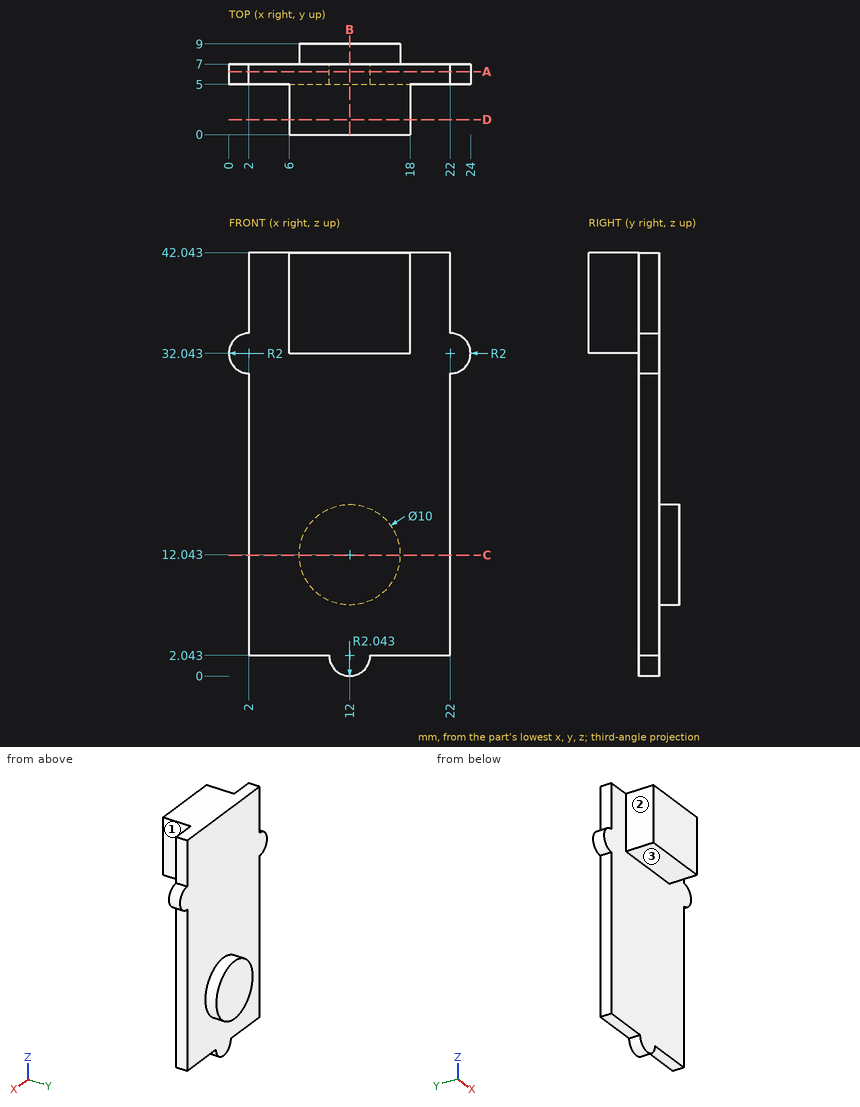
Input: dimensioned drawing with shaded views. Units: mm. Origin: part minimum x, y, z. A direction names the side the tool comes from. Give positions to 0.01 mm unless a question says otherwise; leave off trailing zeros. Loops run counter-clockwise (first coordinate to the right, second up) from the corner with the lowest first, then second, coordinate; pieces in that order, holes last. Notation, with made-up numbers: M -34.5,0.5 L -5.5,0.5 A19 ccw -5.5,5.5 Z; hole C 45,-17.75 d10. An arc over 180 degrees is marked long. Put each result on its own line as item: value.
1) Cut plane A-A, the plane y = 6.25. Return the cut outline in (x, z).
Computed values:
outline: M 2,2.04 L 9.96,2.04 A2.04 ccw 14.04,2.04 L 22,2.04 L 22,30.04 A2 ccw 22,34.04 L 22,42.04 L 2,42.04 L 2,34.04 A2 ccw 2,30.04 Z
2) First-contact query: P1, Ø2, axis at y = 6, z = 14.5, coming from the -X side; P2, Ø2.5, axis at x = 9.5, y = 2.5, coming from the -Z side; P3, Ø1.5, axis at y = 2, z = 36.5, coming from the +X side; P4, Ø12, axis at x = 8.5, z = 19, coming from the +Y side. Flat tips, straight axial feed; report the tip coordinate or a pass-through.
Computed values:
P1: stops at x = 2
P2: stops at z = 32.04
P3: stops at x = 18
P4: stops at y = 9
3) Cut plane C-C, the plane z = 12. Return the cut outline in (x, y).
Computed values:
outline: M 2,5 L 22,5 L 22,7 L 17,7 L 17,9 L 7,9 L 7,7 L 2,7 Z
4) Reachability of the marked faces 1, 2 and 3 from +Z, -Z, +X, -X, +Y, -Y: full face, straight path, thin tool, end or side. Return the list, or none.
Computed values:
face 1: +Z, -Z, +X, -Y
face 2: +Z, -Z, -X, -Y
face 3: -Z, +X, -X, -Y
5) Material intervals for L1, parallel to Y at x = 17.5, z = 26; L2, parallel to X at y = 5.75, z = 15.5; L3, parallel to Z at x = 15, y = 1.5, sorted ascending. Write a range as from..to.
Computed values:
L1: y = 5..7
L2: x = 2..22
L3: z = 32.04..42.04
6) Cut plane B-B, the plane x = 12. Return the cut outline in (y, z), plus the area to 3 significant figures.
Computed values:
outline: M 0,32.04 L 5,32.04 L 5,0 L 7,0 L 7,7.04 L 9,7.04 L 9,17.04 L 7,17.04 L 7,42.04 L 0,42.04 Z
area: 154 mm^2
7) Cut plane D-D, the plane y = 1.5. Return the cut outline in (x, z).
Computed values:
outline: M 6,32.04 L 18,32.04 L 18,42.04 L 6,42.04 Z
